Part model, mm, in its own coordinate system. Round coordinates to 2 decimals unless told otherwise and drop trailing zeros. Loops run counter-clockwise (first coordinate to the right, second up) from the corner with the lowest first, then second, coordinate; pieces in that order, holes last.
1) Band-saw the part on A-A, the plane z = 0. Write the cut outline in (x, y), then the cut area to 3 significant figures.
2) Band-saw the part on C-C, the plane z = -45. Write the cut outline in (x, y), then the cut area to 3 significant figures.
3) Probe line 1 (X direction, y = 2.1, z = 115); line 2 (Z direction, x = -5, y = 1.85); line 3 (X direction, y = 0.8, z = -32). List the from-to ranges inside material, lowest first.
4) Band-saw the part on D-D, the plane x = 22.5. Write the cut outline in (y, z), then the cut area to 3 significant figures.
5) Band-saw the part on B-B, the plane y = 1.95. State how many separate pieces and enclosed holes the cut face has, then the cut area to 3 significant figures.
6) Drop flat-ended pins along their axis: P1, Ø0.9, axis at y = 1, z = -71, coming from the +X side; P2, Ø1.9, axis at x = 0, z = -67, coming from the -Y side (3 decimals); P3, Ø1, axis at x = 18.5, y = 2, coming from the +Z side. Give the stop position or say it passes through.
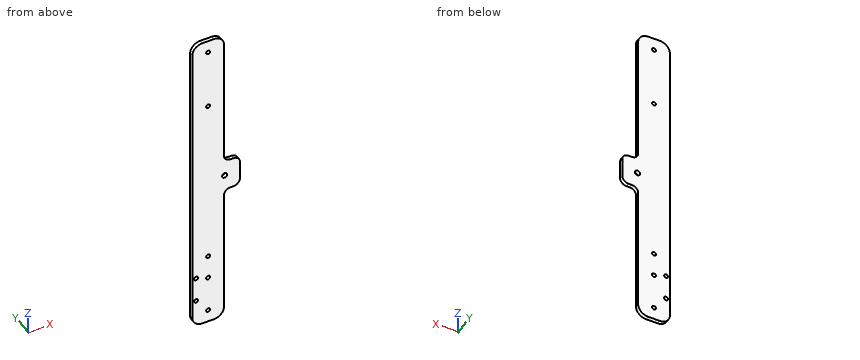
from build123d import *

# Parameters (mm, degrees)
SKETCH_1_W          = 25
SKETCH_1_H          = 250
EXTRUDE_1_DEPTH     = 3
SKETCH_2_R          = 1.55
CUT_EXTRUDE_1_DEPTH = 3
SKETCH_3_R          = 1.55
CUT_EXTRUDE_2_DEPTH = 10
SKETCH_5_W          = 25
SKETCH_5_H          = 25
EXTRUDE_2_DEPTH     = 3
SKETCH_6_R          = 2.05
CUT_EXTRUDE_3_DEPTH = 10
SKETCH_7_R          = 1.55
CUT_EXTRUDE_4_DEPTH = 10
FILLET_1_R          = 5
FILLET_2_R          = 8


with BuildPart() as part:
    # 草图1 → 凸台-拉伸1 (new body)
    with BuildSketch(Plane(origin=(0, 0, 0), x_dir=(1, 0, 0), z_dir=(0, 1, 0))):
        Rectangle(SKETCH_1_W, SKETCH_1_H)
    extrude(amount=EXTRUDE_1_DEPTH)

    # 草图2 → 切除-拉伸1 (cut)
    with BuildSketch(Plane(origin=(0, 0, 0), x_dir=(-1, 0, 0), z_dir=(0, -1, 0))):
        with Locations(Location((0, 115, 0), (0, 0, 90))):
            Circle(SKETCH_2_R)
        with Locations(Location((0, 67, 0), (0, 0, 90))):
            Circle(SKETCH_2_R)
        with Locations(Location((0, -67, 0), (0, 0, 90))):
            Circle(SKETCH_2_R)
        with Locations(Location((0, -115, 0), (0, 0, 90))):
            Circle(SKETCH_2_R)
    extrude(amount=-CUT_EXTRUDE_1_DEPTH, mode=Mode.SUBTRACT)

    # 草图3 → 切除-拉伸2 (cut)
    with BuildSketch(Plane(origin=(0, 0, 0), x_dir=(-1, 0, 0), z_dir=(0, -1, 0))):
        with Locations(Location((9.5, 83, 0), (0, 0, 90))):
            Circle(SKETCH_3_R)
        with Locations(Location((9.5, 103, 0), (0, 0, 90))):
            Circle(SKETCH_3_R)
    extrude(amount=-CUT_EXTRUDE_2_DEPTH, mode=Mode.SUBTRACT)

    # 草图5 → 凸台-拉伸2 (add, through all)
    with BuildSketch(Plane(origin=(0, 0, 0), x_dir=(-1, 0, 0), z_dir=(0, -1, 0))):
        with Locations((-12.5, 0)):
            Rectangle(SKETCH_5_W, SKETCH_5_H)
    extrude(amount=-EXTRUDE_2_DEPTH)

    # 草图6 → 切除-拉伸3 (cut)
    with BuildSketch(Plane(origin=(0, 0, 0), x_dir=(-1, 0, 0), z_dir=(0, -1, 0))):
        with Locations(Location((-13, 0, 0), (0, 0, 90))):
            Circle(SKETCH_6_R)
    extrude(amount=-CUT_EXTRUDE_3_DEPTH, mode=Mode.SUBTRACT)

    # 草图7 → 切除-拉伸4 (cut)
    with BuildSketch(Plane(origin=(0, 0, 0), x_dir=(-1, 0, 0), z_dir=(0, -1, 0))):
        with Locations(Location((0, 86, 0), (0, 0, 90))):
            Circle(SKETCH_7_R)
    extrude(amount=-CUT_EXTRUDE_4_DEPTH, mode=Mode.SUBTRACT)

    # 圆角1
    fillet_1_edges = [part.edges().sort_by_distance(p)[0] for p in [
        (25, 1.5, -12.5),
        (12.5, 1.5, 12.5),
        (25, 1.5, 12.5),
        (12.5, 1.5, -12.5),
    ]]
    fillet(fillet_1_edges, radius=FILLET_1_R)

    # 圆角2
    fillet_2_edges = [part.edges().sort_by_distance(p)[0] for p in [
        (12.5, 1.5, 125),
        (-12.5, 1.5, 125),
        (-12.5, 1.5, -125),
        (12.5, 1.5, -125),
    ]]
    fillet(fillet_2_edges, radius=FILLET_2_R)


solid = part.part
Reported:
1. outline: (-12.5, 0) - (10.95, 0) - (10.95, 3) - (-12.5, 3) - close; (15.05, 0) - (25, 0) - (25, 3) - (15.05, 3) - close
1. area: 100 mm2
2. outline: (-12.5, 0) - (12.5, 0) - (12.5, 3) - (-12.5, 3) - close
2. area: 75.0 mm2
3. line 1: x = -12.5 to -1.55, 1.55 to 12.5
3. line 2: z = -124.98 to 124.98
3. line 3: x = -12.5 to 12.5
4. outline: (0, -11.83) - (3, -11.83) - (3, 11.83) - (0, 11.83) - close
4. area: 71.0 mm2
5. separate pieces: 1
5. enclosed holes: 8
5. area: 6,440 mm2
6. P1: stops at x = 12.5
6. P2: passes through
6. P3: stops at z = 12.5
